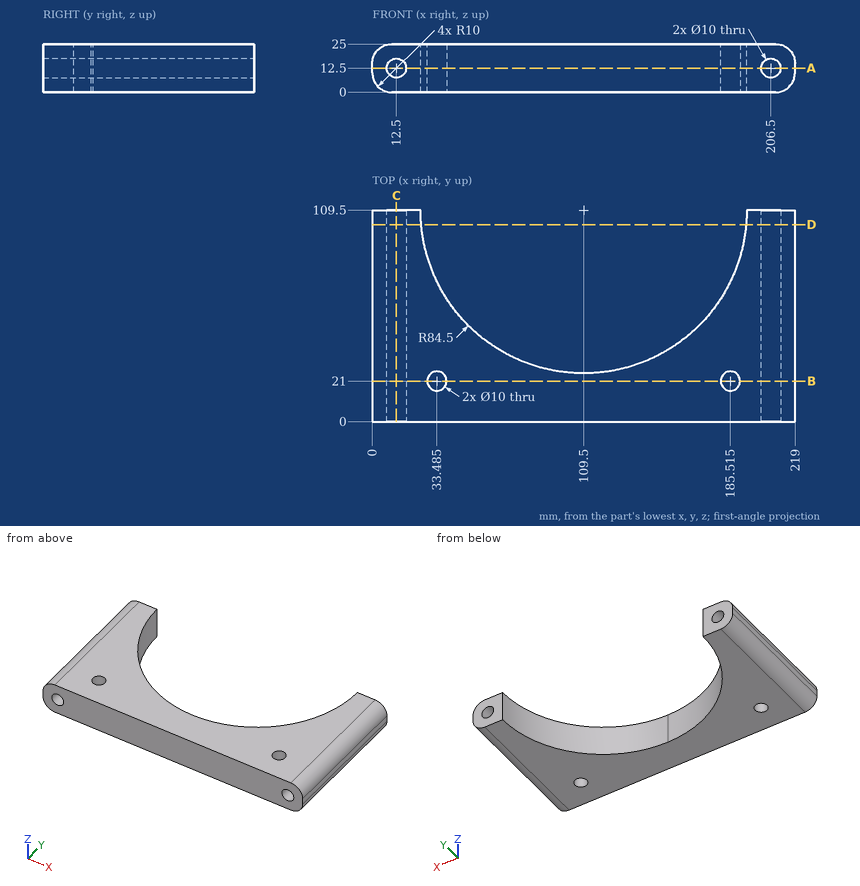
Job drawing, mm, ordinate dimensions from the low corner. One solid piece. Round coordinates to 2 decimals unless told otherwise and drop trailing zeros. Order: outer loops, then holes, each group sorted by start corner. A loop starts at its lowest first (then second) coordinate and runs counter-clockwise, first axis right, second up. Notation, with made-up numbers: (-12, -19.5) -> (-8, -19.5) arc R28 ccw to (-8, 13.5) -> close; hole circle Ø6 at (-33.5, 50). An arc over 180 degrees is marked (long way). Answer in a Markdown table with one row per item.
1) Band-saw the part on C-C on x = 12.5. Give the cut face in (y, z).
Values:
| item | result |
|---|---|
| outline | (0, 0) -> (109.5, 0) -> (109.5, 7.5) -> (0, 7.5) -> close; (0, 17.5) -> (109.5, 17.5) -> (109.5, 25) -> (0, 25) -> close |
2) Wall check: L1, parallel to X at y = 24.5, z = 5.5; L2, parallel to X at y = 41, z = 16.25; L3, parallel to X at y = 41, z = 12.75. Give the ranges that are in metal, low to high.
Values:
| item | result |
|---|---|
| L1 | 1.07 to 29.91, 37.06 to 181.94, 189.09 to 217.93 |
| L2 | 0.08 to 9.19, 15.81 to 60.02, 158.98 to 203.19, 209.81 to 218.92 |
| L3 | 0 to 7.51, 17.49 to 60.02, 158.98 to 201.51, 211.49 to 219 |
3) Band-saw the part on A-A on z = 12.5. Give the cut face in (x, y) (3 decimals), and give its area (3 significant figures).
Values:
| item | result |
|---|---|
| outline | (0, 0) -> (7.5, 0) -> (7.5, 109.5) -> (0, 109.5) -> close; (17.5, 0) -> (201.5, 0) -> (201.5, 109.5) -> (194, 109.5) arc R84.5 cw to (25, 109.5) -> (17.5, 109.5) -> close; (211.5, 0) -> (219, 0) -> (219, 109.5) -> (211.5, 109.5) -> close; hole circle Ø10 at (33.485, 21); hole circle Ø10 at (185.515, 21) |
| area | 10,400 mm2 |
4) Band-saw the part on B-B on y = 21. Give the cut face in (x, z) (3 decimals), and give its area (3 significant figures).
Values:
| item | result |
|---|---|
| outline | (0, 10) arc R10 ccw to (10, 0) -> (28.485, 0) -> (28.485, 25) -> (10, 25) arc R10 ccw to (0, 15) -> close; (38.485, 0) -> (180.515, 0) -> (180.515, 25) -> (38.485, 25) -> close; (190.515, 0) -> (209, 0) arc R10 ccw to (219, 10) -> (219, 15) arc R10 ccw to (209, 25) -> (190.515, 25) -> close; hole circle Ø10 at (12.5, 12.5); hole circle Ø10 at (206.5, 12.5) |
| area | 4,730 mm2 |
5) Pin check, flat tips, straight feed: P1, Ø8, axis at y = 27.5, z = 9.5, coming from the -X side; P2, Ø1, axis at y = 15.5, z = 4.5, coming from the -X side; P3, Ø4, axis at x = 33.5, z = 16, coming from the +Y side. Stop position of each tip, or through.
Values:
| item | result |
|---|---|
| P1 | x = 0 |
| P2 | x = 1.34 |
| P3 | y = 77 |
6) Band-saw the part on D-D on y = 102. Give the cut face in (x, z).
Values:
| item | result |
|---|---|
| outline | (0, 10) arc R10 ccw to (10, 0) -> (25.33, 0) -> (25.33, 25) -> (10, 25) arc R10 ccw to (0, 15) -> close; (193.67, 0) -> (209, 0) arc R10 ccw to (219, 10) -> (219, 15) arc R10 ccw to (209, 25) -> (193.67, 25) -> close; hole circle Ø10 at (12.5, 12.5); hole circle Ø10 at (206.5, 12.5) |
